The listing builds one solid part. Answer for the finished solid, in the listing's coordinates (mm). Round coordinates to 2 decimals unless told otherwise and drop trailing zeros. Order: outer loops, then holes, each group sorted by start corner. A loop starts at its lowest first (then second) coordinate and runs counter-clockwise, first axis right, second up. Notation, with made-up numbers: M 48.25,55.5 L 55.25,55.5 A23 cw 55.25,66.5 Z; hole C 17.5,-40 d1. An arc over 180 degrees is marked long. Put each result on its own line as item: value. Start each with the question number.
1. Consider line 1 (Z direction, x = 15, y = -241); line 2 (Z direction, x = 65, y = -85.5). Determine where each line is inside the solid, lowest interval first.
2. The part is cut by section C-C (y = -213). Give the vertices of the cut face in (x, z), then the cut area to 3 significant figures.
3. The mould has two halves that part along Y. Classify faces 1 (the face through (-15.65, -148.63, 6)), 2 (the face through (-88.95, -148, 5)), 3 (the face through (-84.67, -295.49, 4.93)): +Y half, -Y half, draft (parallel to the pull), parting line (faces both ways), or undercut.
4. The part is cut by section A-A (y = -125). Give the vertices of the cut face in (x, z).
5. The part is cut by section B-B (x = 54.5). Give the vertices of the cut face in (y, z), then the cut area to 3 significant figures.
6. Each of these flat-tipped pins is pushed along its axis until it touches: pin 1 Ø1.5 at (x, y) = (74, -118.5) entering from -Z; pin 2 Ø1.5 at (x, y) = (-47.5, -265) entering from +Z. Where does it stop, or does it pass through?
from build123d import *

# Parameters (mm, degrees)
F1_DEPTH     = 300
F2_R         = 15
F4_DEPTH     = 1
F5_T1_DEPTH  = 108.3513065438
F5_T3_DEPTH  = 259.0557519346
F5_T5_DEPTH  = 108.3513065438
F5_T8_ANGLE  = 90
F5_T10_ANGLE = 90
F5_T12_ANGLE = 90
F5_T14_ANGLE = 90
F7_DEPTH     = 0.1
F9_DEPTH     = 1


# Not quite as in the source:
# - a fillet or chamfer that OpenCascade refuses, or shapes differently, is made with other operations: its cross-section is extruded or revolved along the edge and cut away or added


with BuildPart() as f1:
    # F0 (on Front) → F1 (new body)
    with BuildSketch(Plane.XZ):
        Polygon((-88.9504104853, 0), (131.0495895147, 0), (131.0495895147, 1), (-88.9504104853, 10), align=None)
    extrude(amount=F1_DEPTH)

    # F2
    f2_edges = [f1.edges().sort_by_distance(p)[0] for p in [
        (-88.95041, -300, 5),
        (131.04959, -300, 0.5),
        (131.04959, 0, 0.5),
        (-88.95041, 0, 5),
    ]]
    fillet(f2_edges, radius=F2_R)

    # F3 (on face) → F4 (cut)
    with BuildSketch(Plane(origin=(0.2597928415, 0, 6.3504916821), x_dir=(0.999164272, 0, -0.040874902), z_dir=(0.040874902, 0, 0.999164272))):
        with BuildLine():
            ThreePointArc((-74.2722747486, -280), (-72.8078086545, -283.5355339059), (-69.2722747486, -285))
            Line((-69.2722747486, -285), (39.0790317953, -285))
            ThreePointArc((39.0790317953, -285), (42.6145657012, -283.5355339059), (44.0790317953, -280))
            Line((44.0790317953, -280), (44.0790317953, -20.9442480654))
            ThreePointArc((44.0790317953, -20.9442480654), (42.6145657012, -17.4087141594), (39.0790317953, -15.9442480654))
            Line((39.0790317953, -15.9442480654), (-69.2722747486, -15.9442480654))
            ThreePointArc((-69.2722747486, -15.9442480654), (-72.8078086545, -17.4087141594), (-74.2722747486, -20.9442480654))
            Line((-74.2722747486, -20.9442480654), (-74.2722747486, -280))
        make_face()
    extrude(amount=-F4_DEPTH, mode=Mode.SUBTRACT)

    # F5: fillet of radius 5 on 8 edges, made by hand

    # F5_s2 → F5_t1 (join)
    with BuildSketch(Plane(origin=(-69.214381967, 0, 2.8314974441), x_dir=(0, 1, 0), z_dir=(0.999164272, 0, -0.040874902))):
        with BuildLine():
            ThreePointArc((-285, 6.3558034051), (-283.5811388301, 5.6123869149), (-282, 5.3558034051))
            Line((-282, 5.3558034051), (-285, 5.3558034051))
            Line((-285, 5.3558034051), (-285, 6.3558034051))
        make_face()
    extrude(amount=F5_T1_DEPTH)

    # F5_s4 → F5_t3 (join)
    with BuildSketch(Plane.XZ.offset(20.9442480654)):
        with BuildLine():
            ThreePointArc((44.3019865544, 4.5487655756), (42.8539240904, 3.8639661907), (41.2636188365, 3.6722260098))
            Line((41.2636188365, 3.6722260098), (44.2611116524, 3.5496013037))
            Line((44.2611116524, 3.5496013037), (44.3019865544, 4.5487655756))
        make_face()
        with BuildLine():
            ThreePointArc((-73.9504104853, 9.3863636364), (-72.5631221736, 8.5855726288), (-70.9937925714, 8.2645746583))
            Line((-70.9937925714, 8.2645746583), (-73.9912853873, 8.3871993644))
            Line((-73.9912853873, 8.3871993644), (-73.9504104853, 9.3863636364))
        make_face()
    extrude(amount=F5_T3_DEPTH)

    # F5_s6 → F5_t5 (join)
    with BuildSketch(Plane(origin=(39.0463723531, 0, -1.5973515963), x_dir=(0, 1, 0), z_dir=(-0.999164272, 0, 0.040874902))):
        with BuildLine():
            ThreePointArc((-15.9442480654, -6.3558034051), (-17.3631092353, -5.6123869149), (-18.9442480654, -5.3558034051))
            Line((-18.9442480654, -5.3558034051), (-15.9442480654, -5.3558034051))
            Line((-15.9442480654, -5.3558034051), (-15.9442480654, -6.3558034051))
        make_face()
    extrude(amount=F5_T5_DEPTH)

    # F5_s7 → F5_t8 (revolve)
    with BuildSketch(Plane.XZ.offset(280)):
        with BuildLine():
            ThreePointArc((-73.9504104853, 9.3863636364), (-72.5631221736, 8.5855726288), (-70.9937925714, 8.2645746583))
            Line((-70.9937925714, 8.2645746583), (-73.9912853873, 8.3871993644))
            Line((-73.9912853873, 8.3871993644), (-73.9504104853, 9.3863636364))
        make_face()
    revolve(axis=Axis((-68.9954640274, -280, 8.1828248542), (0.040874902, 0, 0.999164272)), revolution_arc=F5_T8_ANGLE)

    # F5_s9 → F5_t10 (revolve)
    with BuildSketch(Plane(origin=(39.046372353, 0, -1.5973515963), x_dir=(0, 1, 0), z_dir=(-0.999164272, 0, 0.040874902))):
        with BuildLine():
            ThreePointArc((-285, -6.3558034051), (-283.5811388301, -5.6123869149), (-282, -5.3558034051))
            Line((-282, -5.3558034051), (-285, -5.3558034051))
            Line((-285, -5.3558034051), (-285, -6.3558034051))
        make_face()
    revolve(axis=Axis((39.2652902926, -280, 3.7539758139), (0.040874902, 0, 0.999164272)), revolution_arc=F5_T10_ANGLE)

    # F5_s11 → F5_t12 (revolve)
    with BuildSketch(Plane.XZ.offset(20.9442480654)):
        with BuildLine():
            ThreePointArc((44.3019865544, 4.5487655756), (42.8539240904, 3.8639661907), (41.2636188365, 3.6722260098))
            Line((41.2636188365, 3.6722260098), (44.2611116524, 3.5496013037))
            Line((44.2611116524, 3.5496013037), (44.3019865544, 4.5487655756))
        make_face()
    revolve(axis=Axis((39.2652902926, -20.9442480654, 3.7539758139), (0.040874902, 0, 0.999164272)), revolution_arc=F5_T12_ANGLE)

    # F5_s13 → F5_t14 (revolve)
    with BuildSketch(Plane(origin=(-69.214381967, 0, 2.8314974441), x_dir=(0, 1, 0), z_dir=(0.999164272, 0, -0.040874902))):
        with BuildLine():
            ThreePointArc((-15.9442480654, 6.3558034051), (-17.3631092353, 5.6123869149), (-18.9442480654, 5.3558034051))
            Line((-18.9442480654, 5.3558034051), (-15.9442480654, 5.3558034051))
            Line((-15.9442480654, 5.3558034051), (-15.9442480654, 6.3558034051))
        make_face()
    revolve(axis=Axis((-68.9954640274, -20.9442480654, 8.1828248542), (0.040874902, 0, 0.999164272)), revolution_arc=F5_T14_ANGLE)

    # F6 (on face) → F7 (cut)
    with BuildSketch(Plane(origin=(0.2597928415, 0, 6.3504916821), x_dir=(0.999164272, 0, -0.040874902), z_dir=(0.040874902, 0, 0.999164272))):
        with BuildLine():
            ThreePointArc((117.753483355, -100.5515882969), (117.4605901362, -99.8444815157), (116.753483355, -99.5515882969))
            Line((116.753483355, -99.5515882969), (49.977278173, -99.5515882969))
            ThreePointArc((49.977278173, -99.5515882969), (49.2701713918, -99.8444815157), (48.977278173, -100.5515882969))
            Line((48.977278173, -100.5515882969), (48.977278173, -199.4484117031))
            ThreePointArc((48.977278173, -199.4484117031), (49.2701713918, -200.1555184843), (49.977278173, -200.4484117031))
            Line((49.977278173, -200.4484117031), (116.753483355, -200.4484117031))
            ThreePointArc((116.753483355, -200.4484117031), (117.4605901362, -200.1555184843), (117.753483355, -199.4484117031))
            Line((117.753483355, -199.4484117031), (117.753483355, -100.5515882969))
        make_face()
    extrude(amount=-F7_DEPTH, mode=Mode.SUBTRACT)

    # F8 (on face) → F9 (join)
    with BuildSketch(Plane(origin=(0.2189179395, 0, 5.3513274101), x_dir=(0.999164272, 0, -0.040874902), z_dir=(0.040874902, 0, 0.999164272))):
        with BuildLine():
            ThreePointArc((-67.5527229905, -276.7879536152), (-67.4062763811, -277.1415070058), (-67.0527229905, -277.2879536152))
            Line((-67.0527229905, -277.2879536152), (-59.0665953457, -277.2879536152))
            ThreePointArc((-59.0665953457, -277.2879536152), (-58.7130419551, -277.1415070058), (-58.5665953457, -276.7879536152))
            Line((-58.5665953457, -276.7879536152), (-58.5665953457, -264.596647501))
            ThreePointArc((-58.5665953457, -264.596647501), (-58.7130419551, -264.2430941104), (-59.0665953457, -264.096647501))
            Line((-59.0665953457, -264.096647501), (-67.0527229905, -264.096647501))
            ThreePointArc((-67.0527229905, -264.096647501), (-67.4062763811, -264.2430941104), (-67.5527229905, -264.596647501))
            Line((-67.5527229905, -264.596647501), (-67.5527229905, -276.7879536152))
        make_face()
    extrude(amount=F9_DEPTH)


solid = f1.part
Resolved:
1. line 1: 0 to 4.75
1. line 2: 0 to 3.7
2. outline: M -88.95,0 L 131.05,0 L 131.05,1 L 44.3,4.55 A5 cw 41.26,3.67 L -70.99,8.26 A5 cw -73.95,9.39 L -88.95,10 Z
2. area: 1,090 mm2
3. face 1: undercut
3. face 2: draft
3. face 3: -Y half
4. outline: M -88.95,0 L 131.05,0 L 131.05,1 L 117.91,1.54 L 117.91,1.44 L 49.19,4.25 L 49.2,4.35 L 44.3,4.55 A5 cw 41.26,3.67 L -70.99,8.26 A5 cw -73.95,9.39 L -88.95,10 Z
5. outline: M -300,0 L 0,0 L 0,4.13 L -99.55,4.13 L -99.55,4.03 L -200.45,4.03 L -200.45,4.13 L -300,4.13 Z
5. area: 1,230 mm2
6. pin 1: z = 0
6. pin 2: z = 7.33
